```python
from build123d import *

# Parameters (mm, degrees)
F0_W     = 40.64
F0_H     = 40.64
F0_W_2   = 17.78
F1_DEPTH = 25.4
F2_DEPTH = 25.4
F3_W     = 25.4
F3_H     = 15.24
F4_DEPTH = 50.8


with BuildPart() as f1:
    # F0 (on Right) → F1 (new body)
    with BuildSketch(Plane.YZ):
        with Locations((-32.078979, 27.665098)):
            Rectangle(F0_W, F0_H)
        with Locations((-61.288979, 27.665098)):
            Rectangle(F0_W_2, F0_H)
    extrude(amount=-F1_DEPTH)

    # F0 (on Right) → F2 (join)
    with BuildSketch(Plane.YZ):
        with Locations((-61.288979, 27.665098)):
            Rectangle(F0_W_2, F0_H)
    extrude(amount=F2_DEPTH)

    # F3 (on face) → F4 (join)
    with BuildSketch(Plane(origin=(0, 0, 7.345098), x_dir=(1, 0, 0), z_dir=(0, 0, -1))):
        with Locations((-12.7, 44.778979)):
            Rectangle(F3_W, F3_H)
    extrude(amount=F4_DEPTH)


solid = f1.part
```
Geometry check sheet. Reference: the model listing, model coordinates, mm. A direction names the side the tool comes from. Coordinates: 2 decimals unless noted, no trailing zeros. Loops run counter-clockwise (first coordinate to the right, second up) from the corner with the lowest first, then second, coordinate; pieces in that order, holes last.
Item 1: Sectioned sample at D-D, the plane y = -47.5. Record the boundary of the cut face in (x, z).
Item 2: Sectioned sample at C-C, the plane z = 27.5. Record the boundary of the cut face in (x, y).
Item 3: Go/stop test with flat-tipped pins: pin 1 Ø4 at (x, z) = (13, 35) entering from +Y; pin 2 Ø20.5 at (x, z) = (-16.5, -8) entering from +Y; pin 3 Ø10 at (x, y) = (-14.5, -57) entering from -Z; pin 4 Ø14 at (x, y) = (3, -65.5) entering from -Z. Record where each tip stops, or that it passes through.
Item 4: Sectioned sample at B-B, the plane y = -59. Record the boundary of the cut face in (x, z), then the cut area to 3 significant figures.
Item 5: Access from +Z, -Z, +X, -X, +Y, -Y to the whole of each face (thin tool, end or side, straight path). Record for faces 1 (the face through (13, -52.399, 27)), 2 (the face through (-13, -25, 7.345)), 3 (the face through (-13, -52.399, -18)).
Item 6: Thickness scan on line 1 (Z direction, x = -21, y = -37); line 2 (X direction, y = -14.5, z = 7.5); line 3 (Y direction, x = -17.5, z = -21). Record the ranges inside material, lowest first.
Item 7: Sectioned sample at A-A, the plane x = -15. Record the boundary of the cut face in (y, z).
Check result:
1. outline: (-25.4, -43.45) - (0, -43.45) - (0, 47.99) - (-25.4, 47.99) - close
2. outline: (-25.4, -70.18) - (25.4, -70.18) - (25.4, -52.4) - (0, -52.4) - (0, -11.76) - (-25.4, -11.76) - close
3. pin 1: stops at y = -52.4
3. pin 2: stops at y = -37.16
3. pin 3: stops at z = -43.45
3. pin 4: stops at z = 7.35
4. outline: (-25.4, 7.35) - (25.4, 7.35) - (25.4, 47.99) - (-25.4, 47.99) - close
4. area: 2,060 mm2
5. face 1: +Z, -Z, +X, +Y
5. face 2: -Z, +X, -X, +Y
5. face 3: -Z, +X, -X, -Y
6. line 1: z = 7.35 to 47.99
6. line 2: x = -25.4 to 0
6. line 3: y = -52.4 to -37.16
7. outline: (-70.18, 7.35) - (-52.4, 7.35) - (-52.4, -43.45) - (-37.16, -43.45) - (-37.16, 7.35) - (-11.76, 7.35) - (-11.76, 47.99) - (-70.18, 47.99) - close
